Part model, mm, in its own coordinate system. Face numbers are marked on the shaded views. A direction names the side the tool comes from. Give positions to 0.01 mm unless a question says otherwise; leave off trailing zeros. Order: outer loops, then holes, each group sorted by start corner. A loop starts at its lowest first (then second) coordinate and runs counter-clockwise, first axis right, second up.
1. Drop flat-ended pins along their axis: pin 1 Ø3 at (y, z) = (10.5, 49) entering from +X; pin 2 Ø4.5 at (y, z) = (5.5, 0) entering from -X; pin 3 Ø1.5 at (x, y) = (13, 36.5) entering from +Z. Give the stop position or say it passes through.
2. Slice it at C-C on y = 59.5. List the corners of the cut face in (x, z).
3. Probe line 1 (Z direction, x = 14, y = 46.5); line 2 (Y direction, x = 41, z = 3.5). List the from-to ranges inside material, lowest first.
4. Slice it at D-D on y = 26. List the corners of the cut face in (x, z), and give its area (3 significant figures).
5. Which spindle directions (+Z, -Z, +X, -X, +Y, -Y) get a long thin tool onto all of the face, cutting with end or side? Do the marked faces 1, 2, 3 and 4. Say none if no direction does.
6. Mould opens along Z. For the marked faces 5, 6 and 7 say: +Z half, -Z half, draft (parallel to the pull), parting line (faces both ways), or undercut.
7. Slice it at A-A on x = 37.5. List the corners of the cut face in (y, z), and give its area (3 significant figures).
8. Slice it at B-B on z = 13. List the corners of the cut face in (x, y), and give its area (3 significant figures).
from build123d import *

# Parameters (mm, degrees)
F0_W      = 48
F0_H      = 48
F1_DEPTH  = 11.5
F2_W      = 43
F2_H      = 43
F3_DEPTH  = 1
F4_R      = 2
F5_W      = 44.5
F5_H      = 44.5
F6_DEPTH  = 62.4
F7_SIZE   = 5
F9_DEPTH  = 7.15
F11_DEPTH = 44.5
F13_DEPTH = 25
F15_DEPTH = 25


with BuildPart() as f1:
    # F0 (on Front) → F1 (new body)
    with BuildSketch(Plane.XZ):
        with Locations((24, 24)):
            Rectangle(F0_W, F0_H)
    extrude(amount=F1_DEPTH)

    # F2 (on face) → F3 (cut)
    with BuildSketch(Plane.XZ.offset(11.5)):
        with Locations((24, 24)):
            Rectangle(F2_W, F2_H)
    extrude(amount=-F3_DEPTH, mode=Mode.SUBTRACT)

    # F4
    f4_edges = [f1.edges().sort_by_distance(p)[0] for p in [
        (0, -5.75, 48),
        (48, -5.75, 48),
        (48, -5.75, 0),
        (0, -5.75, 0),
    ]]
    fillet(f4_edges, radius=F4_R)

    # F5 (on face) → F6 (join)
    with BuildSketch(Plane(origin=(0, 0, 0), x_dir=(-1, 0, 0), z_dir=(0, 1, 0))):
        with Locations((-24, 24)):
            Rectangle(F5_W, F5_H)
    extrude(amount=F6_DEPTH)

    # F7
    f7_edges = [f1.edges().sort_by_distance(p)[0] for p in [
        (46.25, 31.2, 46.25),
        (1.75, 31.2, 46.25),
        (46.25, 31.2, 1.75),
        (1.75, 31.2, 1.75),
    ]]
    chamfer(f7_edges, length=F7_SIZE)

    # F8 (on face) → F9 (join)
    with BuildSketch(Plane(origin=(0, 62.4, 0), x_dir=(-1, 0, 0), z_dir=(0, 1, 0))):
        Polygon((-4.95, 8.075483), (-4.95, 39.924517), (-8.075483, 43.05), (-39.924517, 43.05), (-43.05, 39.924517), (-43.05, 8.075483), (-39.924517, 4.95), (-8.075483, 4.95), align=None)
    extrude(amount=F9_DEPTH)

    # F10 (on face) → F11 (join, through all)
    with BuildSketch(Plane.YZ.offset(46.25)):
        with BuildLine():
            Line((20, 43.25), (20, 41.25))
            Line((20, 41.25), (28, 41.25))
            Line((28, 41.25), (28, 46.25))
            Line((28, 46.25), (20, 46.25))
            Line((20, 46.25), (17.004263, 46.25))
            ThreePointArc((17.004263, 46.25), (11.12186, 47.280701), (5.940328, 50.25))
            Line((5.940328, 50.25), (0.201208, 48.5))
            Line((0.201208, 48.5), (0.201208, 48))
            Line((0.201208, 48), (3.956015, 48))
            Line((3.956015, 48), (5.940328, 48.25))
            ThreePointArc((5.940328, 48.25), (12.551397, 44.572455), (20, 43.25))
        make_face()
        with BuildLine():
            Line((3.956015, 0), (0.201208, 0))
            Line((0.201208, 0), (0.201208, -0.5))
            Line((0.201208, -0.5), (5.940328, -2.25))
            ThreePointArc((5.940328, -2.25), (11.12186, 0.719299), (17.004263, 1.75))
            Line((17.004263, 1.75), (20, 1.75))
            Line((20, 1.75), (28, 1.75))
            Line((28, 1.75), (28, 6.75))
            Line((28, 6.75), (20, 6.75))
            Line((20, 6.75), (20, 4.75))
            ThreePointArc((20, 4.75), (12.551397, 3.427545), (5.940328, -0.25))
            Line((5.940328, -0.25), (3.956015, 0))
        make_face()
    extrude(amount=-F11_DEPTH)

    # F12 (on face) → F13 (cut)
    with BuildSketch(Plane.XY.offset(46.25)):
        Polygon((41.25, 17.004263), (41.25, 28), (24, 28), (6.75, 28), (6.75, 17.004263), (5.75, 17.004263), (5.75, 0), (6.75, 0), (41.25, 0), (42.25, 0), (42.25, 17.004263), align=None)
    extrude(amount=F13_DEPTH, mode=Mode.SUBTRACT)

    # F14 (on face) → F15 (cut)
    with BuildSketch(Plane(origin=(0, 0, 1.75), x_dir=(1, 0, 0), z_dir=(0, 0, -1))):
        Polygon((41.25, -17.004263), (42.25, -17.004263), (42.25, 0), (41.25, 0), (6.75, 0), (5.75, 0), (5.75, -17.004263), (6.75, -17.004263), (6.75, -28), (41.25, -28), align=None)
    extrude(amount=F15_DEPTH, mode=Mode.SUBTRACT)


solid = f1.part
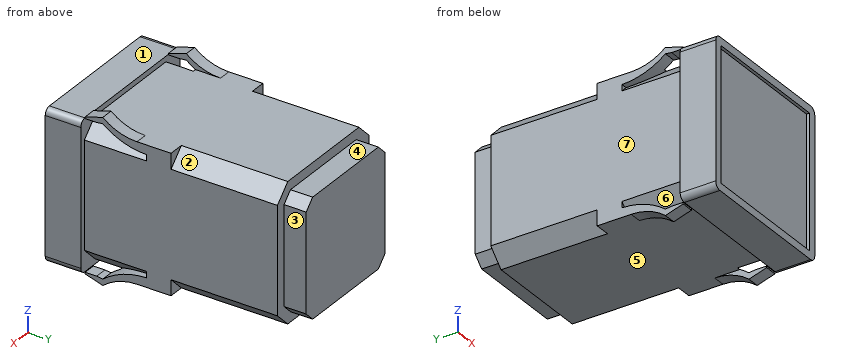
Data:
1. pin 1: stops at x = 46.25
1. pin 2: stops at x = 1.75
1. pin 3: stops at z = 46.25
2. outline: (1.75, 6.75) - (6.75, 1.75) - (41.25, 1.75) - (46.25, 6.75) - (46.25, 41.25) - (41.25, 46.25) - (6.75, 46.25) - (1.75, 41.25) - close
3. line 1: z = 1.75 to 46.25
3. line 2: y = -10.5 to 62.4
4. outline: (1.75, 1.75) - (46.25, 1.75) - (46.25, 46.25) - (1.75, 46.25) - close
4. area: 1,980 mm2
5. face 1: +Z, +X, -X, -Y
5. face 2: +Z, +X, +Y
5. face 3: +Z, -Z, +X, +Y
5. face 4: +Z, +X, -X, +Y
6. face 5: -Z half
6. face 6: undercut
6. face 7: draft
7. outline: (-11.5, 0) - (0, 0) - (0, 1.75) - (62.4, 1.75) - (62.4, 4.95) - (69.55, 4.95) - (69.55, 43.05) - (62.4, 43.05) - (62.4, 46.25) - (0, 46.25) - (0, 48) - (-11.5, 48) - (-11.5, 45.5) - (-10.5, 45.5) - (-10.5, 2.5) - (-11.5, 2.5) - close
7. area: 3,560 mm2
8. outline: (0, -11.5) - (2.5, -11.5) - (2.5, -10.5) - (45.5, -10.5) - (45.5, -11.5) - (48, -11.5) - (48, 0) - (46.25, 0) - (46.25, 62.4) - (43.05, 62.4) - (43.05, 69.55) - (4.95, 69.55) - (4.95, 62.4) - (1.75, 62.4) - (1.75, 0) - (0, 0) - close
8. area: 3,560 mm2
